Design review of the part built by this model. Coordinates are the model's own, in mm. A direction names the side the tool comes from. Give positions to 0.01 mm unless a question says otherwise; leave off trailing zeros. Loops run counter-clockwise (first coordinate to the right, second up) from the corner with the lowest first, then second, coordinate; pieces in that order, holes last. Notation, with made-up numbers: M -20.5,37.25 L 3.5,37.25 A33 cw 3.5,69.25 Z; hole C 80,-19 d4. An arc over 180 degrees is marked long. Answer as CSV lines item,"result".
```python
from build123d import *

# Parameters (mm, degrees)
F2_R     = 4
F3_DEPTH = 16
F4_R     = 3.5
F5_DEPTH = 10


with BuildPart() as f1:
    # F0 (on Front) → F1 (revolve)
    with BuildSketch(Plane.XZ):
        Polygon((0, 12.5), (0, 0), (210, 0), (210, 12.5), (121.6, 12.5), (121.6, 15), (76, 15), (76, 17.5), (44, 17.5), (44, 20), (25, 20), (25, 12.5), align=None)
    revolve(axis=Axis((106.720138, 0, 0), (1, 0, 0)))

    # F2 (on face) → F3 (cut)
    with BuildSketch(Plane(origin=(0, 0, 0), x_dir=(0, -1, 0), z_dir=(-1, 0, 0))):
        Circle(F2_R)
    extrude(amount=-F3_DEPTH, mode=Mode.SUBTRACT)

    # F4 (on face) → F5 (cut)
    with BuildSketch(Plane.YZ.offset(210)):
        Circle(F4_R)
    extrude(amount=-F5_DEPTH, mode=Mode.SUBTRACT)


solid = f1.part
```
1. We need section D-D, the plane z = -8.5. Write out the cut boundary in (x, y), plus the area to 3 significant figures.
Answer block:
outline,"M 0,-9.17 L 25,-9.17 L 25,-18.1 L 44,-18.1 L 44,-15.3 L 76,-15.3 L 76,-12.36 L 121.6,-12.36 L 121.6,-9.17 L 210,-9.17 L 210,9.17 L 121.6,9.17 L 121.6,12.36 L 76,12.36 L 76,15.3 L 44,15.3 L 44,18.1 L 25,18.1 L 25,9.17 L 0,9.17 Z"
area,"4,870 mm²"
2. The part is to be moulded in two halves that separate along Y. For faces 1 (the flat face through (200, 0, 0)), 2 (the flat face through (0, -3, -3)), 3 (the cylindrical face through (165.181, -3.755, 11.923)), say which applies: pulls with the +Y half, pulls with the -Y half, needs draft (parallel to the pull), parting line crosses it, or undercut.
Answer block:
face 1,"undercut"
face 2,"needs draft"
face 3,"parting line crosses it"
3. For faces 4 (the flat face through (76, -8, -13)), 5 (the cylindrical face through (34.367, 19.524, -4.336)), 6 (the flat face through (16, 0, 0)), list the 3-axis set-ups (+Z, -Z, +X, -X, +Y, -Y) from which the entire face can be reached by the end or side of a thin tool; tool diameter is ignored.
Answer block:
face 4,"+X"
face 5,"+X, -X"
face 6,"-X"
4. For P1, Ø4, axis at x = 161, y = -10, coming from the +Z side; P2, Ø6, axis at x = 61.5, z = -15.5, coming from the +Y side; P3, Ø6.5, axis at y = 0, z = 0, coming from the +X side, all flat-tipped, find the tip position at first contact; note any pin that passes through.
Answer block:
P1,"z = 9.6"
P2,"y = 12.25"
P3,"x = 200"
5. We need section C-C, the plane x = 95. Write out the cut boundary in (y, z).
Answer block:
outline,"C 0,0 d30"
6. We need section A-A, the plane z = 0. Write out the cut boundary in (x, y).
Answer block:
outline,"M 0,-12.5 L 25,-12.5 L 25,-20 L 44,-20 L 44,-17.5 L 76,-17.5 L 76,-15 L 121.6,-15 L 121.6,-12.5 L 210,-12.5 L 210,-3.5 L 200,-3.5 L 200,3.5 L 210,3.5 L 210,12.5 L 121.6,12.5 L 121.6,15 L 76,15 L 76,17.5 L 44,17.5 L 44,20 L 25,20 L 25,12.5 L 0,12.5 L 0,4 L 16,4 L 16,-4 L 0,-4 Z"
7. To check wall thickness, follow L1, parallel to Z at x = 9.75, y = 0; L2, parallel to Z at x = 204.75, y = 0; L3, parallel to X at y = 3.5, z = 17. State the ranges of each line that lie inside material, in increasing order. Write a range as [from, to].
Answer block:
L1,"[-12.5, -4], [4, 12.5]"
L2,"[-12.5, -3.5], [3.5, 12.5]"
L3,"[25, 76]"
